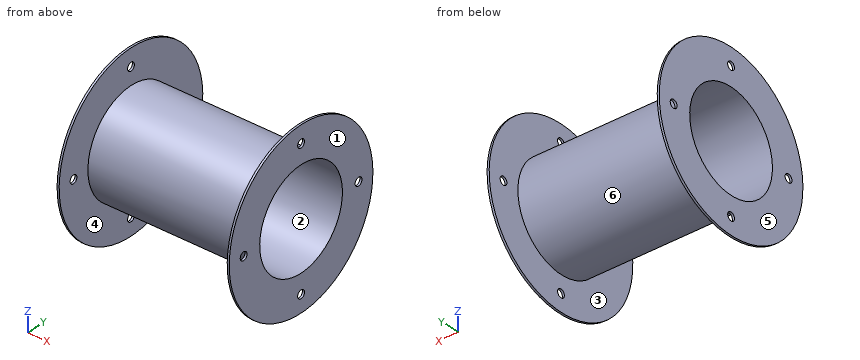
from build123d import *

# Parameters (mm, degrees)
SKETCH4_R          = 3
CUT_EXTRUDE1_DEPTH = 174.713717869
CIRPATTERN1_COUNT  = 4


with BuildPart() as part:
    # Sketch3 → Revolve1 (revolve)
    with BuildSketch(Plane.XY, mode=Mode.PRIVATE) as revolve1_sk:
        Polygon((0, 0), (0, 26.924), (1.524, 26.924), (1.524, 1.524), (125.476, 1.524), (125.476, 26.924), (127, 26.924), (127, 0), align=None)
    revolve(revolve1_sk.sketch.rotate(Axis((-7.37458194, -36.576, 0), (1, 0, 0)), 90), axis=Axis((-7.37458194, -36.576, 0), (1, 0, 0)))

    # Sketch4 → Cut-Extrude1 (cut, symmetric)
    with BuildSketch(Plane.ZY):
        with Locations((0, 14.224)):
            Circle(SKETCH4_R)
    cut_extrude1 = extrude(amount=CUT_EXTRUDE1_DEPTH, both=True, mode=Mode.SUBTRACT)

    # CirPattern1: Cut-Extrude1 ×4 about axis
    cirpattern1_axis = Axis((0, -36.576, 0), (1, 0, 0))
    for i in range(1, CIRPATTERN1_COUNT):
        add(cut_extrude1.rotate(cirpattern1_axis, i * 360 / CIRPATTERN1_COUNT), mode=Mode.SUBTRACT)


solid = part.part
Input: part model. Units: mm. Frame: model coordinates. Face numbers are marked on the shaded views. A direction names the side the tool comes from. Coordinates: 2 decimals unless noted, no trailing zeros. Order: outer loops, then holes, each group sorted by start corner. A loop starts at its lowest first (then second) coordinate and runs counter-clockwise, first axis right, second up.
1. Cut plane C-C, the plane z = 50.8. Return loops of the section in (x, y), plus the area to 3 significant figures.
Checked values:
outline: (0, -74.68) - (1.52, -74.68) - (1.52, -39.58) - (0, -39.58) - close; (0, -33.58) - (1.52, -33.58) - (1.52, 1.52) - (0, 1.52) - close; (125.48, -74.68) - (127, -74.68) - (127, -39.58) - (125.48, -39.58) - close; (125.48, -33.58) - (127, -33.58) - (127, 1.52) - (125.48, 1.52) - close
area: 214 mm2
2. Access query for the marked faces 5 and 6. Directions: +Z, -Z, +X, -X, +Y, -Y. A direction counts if a zero-diameter tool reaches every point of the face in a straight line with its end or side. Return the directions, or none.
Checked values:
face 5: +Z, -Z, -X, +Y, -Y
face 6: none
3. Cut plane D-D, the plane x = 36. Return loops of the section in (y, z).
Checked values:
outline: circle Ø76.2 at (-36.58, 0); hole circle Ø73.15 at (-36.58, 0)
4. Draft query along X for the marked faces 1, 2, 3 and 4. Return one class per face: +X half, -X half, draft (parallel to the pull), parting line (faces both ways), or undercut.
Checked values:
face 1: +X half
face 2: draft
face 3: undercut
face 4: undercut
5. Cut plane B-B, the plane y = -69. Return loops of the section in (x, z), plus the area to 3 significant figures.
Checked values:
outline: (0, -54.6) - (1.52, -54.6) - (1.52, -20.01) - (125.48, -20.01) - (125.48, -54.6) - (127, -54.6) - (127, -16.93) - (0, -16.93) - close; (0, 16.93) - (127, 16.93) - (127, 54.6) - (125.48, 54.6) - (125.48, 20.01) - (1.52, 20.01) - (1.52, 54.6) - (0, 54.6) - close
area: 994 mm2
6. Contact query for flat-ended pins moving along their axis: P1, Ø10, axis at x = 19.5, y = -60, coming from the +Z side; P2, Ø8, axis at x = 39.5, y = -21, coming from the -Z side; P3, Ø3, axis at x = 55.5, y = -11, coming from the +Z side. Output: stop coordinate, or through.
Checked values:
P1: stops at z = 33.35
P2: stops at z = -36.3
P3: stops at z = 29.53
7. Cut plane A-A, the plane z = 0. Count the separate pieces of the cut face and the enclosed holes in it, plus the area to 3 significant figures.
Checked values:
separate pieces: 6
enclosed holes: 0
area: 505 mm2
8. Ray query, line 1 along Y through (x, z) = (126.1, 0); line 2 along X through (y, z) = (-68, -42.5); line 3 along Z through (x, y) = (116.5, -17.5). Return the intervals inside material, ascending.
Checked values:
line 1: y = -100.08 to -90.38, -84.38 to -73.15, 0 to 11.22, 17.22 to 26.92
line 2: x = 0 to 1.52, 125.48 to 127
line 3: z = -32.98 to -31.21, 31.21 to 32.98
